Input: part model. Units: mm. Frame: model coordinates. A direction names the side the tool comes from. Round coordinates to 2 decimals unless told otherwise and drop trailing zeros. Loops run counter-clockwise (first coordinate to the right, second up) from the corner with the lowest first, then second, coordinate; pieces in that order, holes last. Notation, with made-up numbers: M -25,57.25 L -9,57.25 A17 ccw -9,65.25 Z; hole C -25.75,76 d4. An arc over 180 degrees is marked long. Return JSON: item names as keys, results as strings. Group by question number.
1) Mould query, pull axis X, two halves, no side actions, for faces 3 (the face through (210, 30, 5)), 4 (the face through (67, 33, 4.7)), 5 (the face through (6, 7, 5)), 6 (the face through (106, 30, 0)). Classes: +X half, -X half, draft (parallel to the pull), parting line (faces both ways), or undercut.
2) Material intervals for line 1 (Y direction, x = 67.5, z = 7.3); line 2 (X direction, y = 26.5, z = 6.5); line 3 (X direction, y = 21, z = 6), sorted ascending. Write a range as from..to.
3) Access query for faces 1 (the face through (209, 53, 5)), 2 (the face through (107, 33, 4.7)). Directions: +Z, -Z, +X, -X, +Y, -Y. A direction counts if a zero-diameter tool reaches every point of the face in a straight line with its end or side. Return the directions, or none.
4) Section B-B (z = 6.5). Output: boundary loops of the cut face in (x, y), plus the area to 3 significant figures.
5) Contact query for flat-ended pins moving along their axis: P1, Ø1, axis at x = 80.5, y = 40.5, coming from the -Z side; P2, Ø17.5, axis at x = 25.5, y = 27, coming from the +Z side. Output: stop coordinate, or through.
6) Section A-A (x = 67.5). Output: boundary loops of the cut face in (y, z), plus the area to 3 significant figures.
Autodesk Fusion 360 part; units mm, degrees
sketch "Sketch1" plane through (0, 0, 0) normal (0, 0, 1) x (1, 0, 0)
  line L0 (0, 0) -> (235, 0)
  line L1 (235, 0) -> (235, 55)
  line L2 (235, 55) -> (0, 55)
  line L3 (0, 55) -> (0, 0)
  circle A0 centre (27.5, 32.5) radius 17.5
  circle A1 centre (67.5, 32.5) radius 17.5
  circle A2 centre (107.5, 32.5) radius 17.5
  circle A3 centre (147.5, 32.5) radius 17.5
  circle A4 centre (187.5, 32.5) radius 17.5
  dimension "d1" = 235
  dimension "d2" = 55
  dimension "d9" = 35
  dimension "d10" = 35
  dimension "d11" = 35
  dimension "d12" = 35
  dimension "d13" = 35
extrude "Extrude1" add sketch "Sketch1" along normal blind 10
extrude "Extrude2" add sketch "Sketch1" along normal blind 4.7 contours A0 | A1 | A2 | A3 | A4
extrude "Extrude3" cut 1 faces at (235, 18.3333, 3.3333) along direction (-1, 0, 0) blind 20
extrude "Extrude4" cut 1 faces at (215, 18.3333, 3.3333) along direction (-1, 0, 0) blind 5
extrude "Extrude5" cut 1 faces at (0, 36.6667, 3.3333) along direction (1, 0, 0) blind 5
extrude "Extrude6" cut 1 faces at (73.3333, 0, 3.3333) along direction (0, 1, 0) blind 5
fillet "Fillet3" radius 1 5 edges at (11.1843, 38.8283, 10) (51.1843, 38.8283, 10) (91.1843, 38.8283, 10) (131.1843, 38.8283, 10) (171.1843, 38.8283, 10)
fillet "Fillet4" radius 5 4 edges at (210, 5, 5) (5, 5, 5) (5, 55, 5) (210, 55, 5)
Returned:
{
 "1": {"face 3": "+X half", "face 4": "undercut", "face 5": "-X half", "face 6": "draft"},
 "2": {"line 1": "y = 5..15, 50..55", "line 2": "x = 5..11.06, 43.94..51.06, 83.94..91.06, 123.94..131.06, 163.94..171.06, 203.94..210", "line 3": "x = 5..14.31, 40.69..54.31, 80.69..94.31, 120.69..134.31, 160.69..174.31, 200.69..210"},
 "3": {"face 1": "+Z, -Z, +X, +Y", "face 2": "+Z"},
 "4": {"outline": "M 5,10 A5 ccw 10,5 L 205,5 A5 ccw 210,10 L 210,50 A5 ccw 205,55 L 10,55 A5 ccw 5,50 Z; hole C 27.5,32.5 d35; hole C 67.5,32.5 d35; hole C 107.5,32.5 d35; hole C 147.5,32.5 d35; hole C 187.5,32.5 d35", "area": "5,420 mm^2"},
 "5": {"P1": "stops at z = 0", "P2": "stops at z = 4.7"},
 "6": {"outline": "M 5,0 L 55,0 L 55,10 L 51,10 A1 ccw 50,9 L 50,4.7 L 15,4.7 L 15,9 A1 ccw 14,10 L 5,10 Z", "area": "314 mm^2"}
}
